from build123d import *

# Parameters (mm, degrees)
SKETCH1_R           = 9.525
BOSS_EXTRUDE1_DEPTH = 3.175
SKETCH2_R           = 3.81
SKETCH2_R_2         = 2.54
BOSS_EXTRUDE2_DEPTH = 4.064
SKETCH3_R           = 2.54
SKETCH3_R_2         = 1.143
CUT_EXTRUDE1_DEPTH  = 3.175


with BuildPart() as part:
    # Sketch1 → Boss-Extrude1 (new body)
    with BuildSketch(Plane(origin=(0, 0, 0), x_dir=(1, 0, 0), z_dir=(0, 1, 0))):
        Circle(SKETCH1_R)
    extrude(amount=BOSS_EXTRUDE1_DEPTH)

    # Sketch2 → Boss-Extrude2 (add)
    with BuildSketch(Plane(origin=(0, 0, 0), x_dir=(1, 0, 0), z_dir=(0, 1, 0))):
        Circle(SKETCH2_R)
        Circle(SKETCH2_R_2, mode=Mode.SUBTRACT)
    extrude(amount=-BOSS_EXTRUDE2_DEPTH)

    # Sketch3 → Cut-Extrude1 (cut)
    with BuildSketch(Plane(origin=(0, 0, 0), x_dir=(1, 0, 0), z_dir=(0, 1, 0))):
        Circle(SKETCH3_R)
        with Locations((5.08, 0)):
            Circle(SKETCH3_R_2)
        with Locations((0, 5.08)):
            Circle(SKETCH3_R_2)
        with Locations((-5.08, 0)):
            Circle(SKETCH3_R_2)
        with Locations((0, -5.08)):
            Circle(SKETCH3_R_2)
    extrude(amount=CUT_EXTRUDE1_DEPTH, mode=Mode.SUBTRACT)


solid = part.part
Read the model definition and answer for the solid it produces. Units are mm, in the model's axes. A direction names the side the tool comes from. Coordinates: 2 decimals unless noted, no trailing zeros. Loops run counter-clockwise (first coordinate to the right, second up) from the corner with the lowest first, then second, coordinate; pieces in that order, holes last.
Q1. The mould has two halves that part along Z. Classify faces 1 (the face through (-0.33, -0.5, -2.52)), 2 (the face through (-0.83, -2, 3.72)), 3 (the face through (2, 3.175, 2)): +Z half, -Z half, draft (parallel to the pull), parting line (faces both ways), or undercut.
Q2. Which of the six approach directions +Z, -Z, +X, -X, +Y, -Y give full straight-line access (tool end or side, diameter ignored) to faces 4 (the face through (4, 0, 2)), 5 (the face through (3.94, 1.57, -0.05))?
Q3. The part is cut by section C-C on x = 4.75. Write down the section's boundary in (y, z) (3 decimals).
Q4. Each of these flat-tipped pins is pushed along its axis until it touches: pin 1 Ø1.8 at (x, z) = (0, 5.08) entering from +Y; pin 2 Ø1.5 at (x, y) = (-3, -3) entering from +Z; pin 3 Ø1.5 at (y, z) = (-3, 1.5) entering from -X; pin 4 Ø1 at (x, z) = (-7.5, 2) entering from -Y. Where does it stop, or does it pass through?
Q5. The part is cut by section D-D on z = 5.08. Write down the section's boundary in (x, y) (3 decimals), and give its area (3 significant figures).
Q6. The part is cut by section A-A on z = 0. Write down the section's boundary in (x, y) (3 decimals).
Q7. The part is cut by section B-B on x = 0. Write down the section's boundary in (y, z) (3 decimals).
Q8. Consider probe 1 along X at (y, z) = (1.5, 0) (3 decimals); probe 2 along Z at (x, y) = (0, -2). Determine where each line is inside the solid, lowest interval first.
Results below:
1. face 1: undercut
1. face 2: parting line
1. face 3: draft
2. face 4: -Y
2. face 5: +Y, -Y
3. outline: (0, -8.256) - (3.175, -8.256) - (3.175, -1.094) - (0, -1.094) - close; (0, 1.094) - (3.175, 1.094) - (3.175, 8.256) - (0, 8.256) - close
4. pin 1: passes through
4. pin 2: stops at z = 3.07
4. pin 3: stops at x = -3.74
4. pin 4: stops at y = 0
5. outline: (-8.057, 0) - (-1.143, 0) - (-1.143, 3.175) - (-8.057, 3.175) - close; (1.143, 0) - (8.057, 0) - (8.057, 3.175) - (1.143, 3.175) - close
5. area: 43.9 mm2
6. outline: (-9.525, 0) - (-6.223, 0) - (-6.223, 3.175) - (-9.525, 3.175) - close; (-3.937, 0) - (-3.81, 0) - (-3.81, -4.064) - (-2.54, -4.064) - (-2.54, 3.175) - (-3.937, 3.175) - close; (2.54, -4.064) - (3.81, -4.064) - (3.81, 0) - (3.937, 0) - (3.937, 3.175) - (2.54, 3.175) - close; (6.223, 0) - (9.525, 0) - (9.525, 3.175) - (6.223, 3.175) - close
7. outline: (-4.064, -3.81) - (0, -3.81) - (0, -3.937) - (3.175, -3.937) - (3.175, -2.54) - (-4.064, -2.54) - close; (-4.064, 2.54) - (3.175, 2.54) - (3.175, 3.937) - (0, 3.937) - (0, 3.81) - (-4.064, 3.81) - close; (0, -9.525) - (3.175, -9.525) - (3.175, -6.223) - (0, -6.223) - close; (0, 6.223) - (3.175, 6.223) - (3.175, 9.525) - (0, 9.525) - close
8. probe 1: x = -9.525 to -6.223, -3.937 to -2.54, 2.54 to 3.937, 6.223 to 9.525
8. probe 2: z = -3.81 to -2.54, 2.54 to 3.81
